Verification items for the finished model (mm, model axes). A direction names the side the tool comes from. Give positions to 0.01 mm unless a question says otherwise; leave off trailing zeros. Order: outer loops, then holes, each group sorted by start corner. A loop starts at its lowest first (then second) coordinate and runs counter-clockwise, first axis right, second up.
from build123d import *

# Parameters (mm, degrees)
SKETCH1_W                      = 60
SKETCH1_H                      = 322.5
BASE_FLANGE1_DEPTH             = 3
EDGE_FLANGE1_STRIP_W           = 14
EDGE_FLANGE1_STRIP_H           = 3
EDGE_FLANGE1_STRIP_CUT_DEPTH   = 322.5
EDGE_FLANGE1_DEPTH             = 322.5
EDGE_FLANGE2_STRIP_W           = 14
EDGE_FLANGE2_STRIP_H           = 3
EDGE_FLANGE2_STRIP_CUT_DEPTH   = 56
EDGE_FLANGE2_STRIP_2_W         = 14
EDGE_FLANGE2_STRIP_2_H         = 3
EDGE_FLANGE2_STRIP_CUT_2_DEPTH = 56
EDGE_FLANGE2_STRIP_3_W         = 14
EDGE_FLANGE2_STRIP_3_H         = 3
EDGE_FLANGE2_STRIP_CUT_3_DEPTH = 56
EDGE_FLANGE2_STRIP_4_W         = 14
EDGE_FLANGE2_STRIP_4_H         = 3
EDGE_FLANGE2_STRIP_CUT_4_DEPTH = 56
EDGE_FLANGE2_DEPTH             = 56
EDGE_FLANGE2_BEND_DEPTH        = 56
EDGE_FLANGE2_BEND_2_DEPTH      = 56
EDGE_FLANGE2_BEND_3_DEPTH      = 56
SKETCH18_R                     = 4.6
EXTRUDE1_DEPTH                 = 335.806287277
SKETCH19_R                     = 4.6
EXTRUDE2_DEPTH                 = 3
SKETCH20_R                     = 4.6
EXTRUDE3_DEPTH                 = 3


# Sheet-metal steps are written as plain solids
with BuildPart() as part:
    # Sketch1 → Base-Flange1 (new body)
    with BuildSketch(Plane(origin=(0, 0, 0), x_dir=(1, 0, 0), z_dir=(0, 1, 0))):
        Rectangle(SKETCH1_W, SKETCH1_H)
    extrude(amount=BASE_FLANGE1_DEPTH)

    # Edge-Flange1 strip (across the edge) → Edge-Flange1 strip cut (cut)
    with BuildSketch(Plane(origin=(-30, 3, -161.25), x_dir=(1, 0, 0), z_dir=(0, 0, 1))):
        with Locations((-3, -1.5)):
            Rectangle(EDGE_FLANGE1_STRIP_W, EDGE_FLANGE1_STRIP_H)
    extrude(amount=EDGE_FLANGE1_STRIP_CUT_DEPTH, mode=Mode.SUBTRACT)

    # Edge-Flange1 section (across the edge) → Edge-Flange1 (add)
    with BuildSketch(Plane(origin=(-30, 3, -161.25), x_dir=(1, 0, 0), z_dir=(0, 0, 1))):
        with BuildLine():
            Line((0, 1), (0, 57))
            Line((0, 57), (3, 57))
            Line((3, 57), (3, 1))
            ThreePointArc((3, 1), (3.292893219, 0.292893219), (4, 0))
            Line((4, 0), (4, -3))
            ThreePointArc((4, -3), (1.171572875, -1.828427125), (0, 1))
        make_face()
    extrude(amount=EDGE_FLANGE1_DEPTH)

    # Edge-Flange2 strip (across the edge) → Edge-Flange2 strip cut (cut)
    with BuildSketch(Plane(origin=(-30, 4, 161.25), x_dir=(0, 0, -1), z_dir=(0, 1, 0))):
        with Locations((-3, -1.5)):
            Rectangle(EDGE_FLANGE2_STRIP_W, EDGE_FLANGE2_STRIP_H)
    extrude(amount=EDGE_FLANGE2_STRIP_CUT_DEPTH, mode=Mode.SUBTRACT)

    # Edge-Flange2 strip 2 (across the edge) → Edge-Flange2 strip cut 2 (cut)
    with BuildSketch(Plane(origin=(30, 0, 161.25), x_dir=(0, 0, -1), z_dir=(-1, 0, 0))):
        with Locations((-3, -1.5)):
            Rectangle(EDGE_FLANGE2_STRIP_2_W, EDGE_FLANGE2_STRIP_2_H)
    extrude(amount=EDGE_FLANGE2_STRIP_CUT_2_DEPTH, mode=Mode.SUBTRACT)

    # Edge-Flange2 strip 3 (across the edge) → Edge-Flange2 strip cut 3 (cut)
    with BuildSketch(Plane(origin=(-30, 60, -161.25), x_dir=(0, 0, 1), z_dir=(0, -1, 0))):
        with Locations((-3, -1.5)):
            Rectangle(EDGE_FLANGE2_STRIP_3_W, EDGE_FLANGE2_STRIP_3_H)
    extrude(amount=EDGE_FLANGE2_STRIP_CUT_3_DEPTH, mode=Mode.SUBTRACT)

    # Edge-Flange2 strip 4 (across the edge) → Edge-Flange2 strip cut 4 (cut)
    with BuildSketch(Plane(origin=(-26, 0, -161.25), x_dir=(0, 0, 1), z_dir=(1, 0, 0))):
        with Locations((-3, -1.5)):
            Rectangle(EDGE_FLANGE2_STRIP_4_W, EDGE_FLANGE2_STRIP_4_H)
    extrude(amount=EDGE_FLANGE2_STRIP_CUT_4_DEPTH, mode=Mode.SUBTRACT)

    # Edge-Flange2 section (across the edge) → Edge-Flange2 (add)
    with BuildSketch(Plane(origin=(-30, 4, 161.25), x_dir=(0, 0, -1), z_dir=(0, 1, 0))):
        with BuildLine():
            Line((0, 1), (0, 37))
            Line((0, 37), (3, 37))
            Line((3, 37), (3, 1))
            ThreePointArc((3, 1), (3.292893219, 0.292893219), (4, 0))
            Line((4, 0), (4, -3))
            ThreePointArc((4, -3), (1.171572875, -1.828427125), (0, 1))
        make_face()
    extrude(amount=EDGE_FLANGE2_DEPTH)

    # Edge-Flange2 section 2 (across the edge) → Edge-Flange2 bend (add)
    with BuildSketch(Plane(origin=(30, 0, 161.25), x_dir=(0, 0, -1), z_dir=(-1, 0, 0))):
        with BuildLine():
            Line((0, 1), (0, 37))
            Line((0, 37), (3, 37))
            Line((3, 37), (3, 1))
            ThreePointArc((3, 1), (3.292893219, 0.292893219), (4, 0))
            Line((4, 0), (4, -3))
            ThreePointArc((4, -3), (1.171572875, -1.828427125), (0, 1))
        make_face()
    extrude(amount=EDGE_FLANGE2_BEND_DEPTH)

    # Edge-Flange2 section 3 (across the edge) → Edge-Flange2 bend 2 (add)
    with BuildSketch(Plane(origin=(-30, 60, -161.25), x_dir=(0, 0, 1), z_dir=(0, -1, 0))):
        with BuildLine():
            Line((0, 1), (0, 37))
            Line((0, 37), (3, 37))
            Line((3, 37), (3, 1))
            ThreePointArc((3, 1), (3.292893219, 0.292893219), (4, 0))
            Line((4, 0), (4, -3))
            ThreePointArc((4, -3), (1.171572875, -1.828427125), (0, 1))
        make_face()
    extrude(amount=EDGE_FLANGE2_BEND_2_DEPTH)

    # Edge-Flange2 section 4 (across the edge) → Edge-Flange2 bend 3 (add)
    with BuildSketch(Plane(origin=(-26, 0, -161.25), x_dir=(0, 0, 1), z_dir=(1, 0, 0))):
        with BuildLine():
            Line((0, 1), (0, 37))
            Line((0, 37), (3, 37))
            Line((3, 37), (3, 1))
            ThreePointArc((3, 1), (3.292893219, 0.292893219), (4, 0))
            Line((4, 0), (4, -3))
            ThreePointArc((4, -3), (1.171572875, -1.828427125), (0, 1))
        make_face()
    extrude(amount=EDGE_FLANGE2_BEND_3_DEPTH)

    # Sketch18 → Extrude1 (cut, through all)
    with BuildSketch(Plane.XY.offset(161.25)):
        with Locations((-47, 47.5)):
            Circle(SKETCH18_R)
        with Locations((-47, 17.5)):
            Circle(SKETCH18_R)
        with Locations((-12.5, -17)):
            Circle(SKETCH18_R)
        with Locations((17.5, -17)):
            Circle(SKETCH18_R)
    extrude(amount=-EXTRUDE1_DEPTH, mode=Mode.SUBTRACT)

    # Sketch19 → Extrude2 (cut)
    with BuildSketch(Plane(origin=(-27, 0, 0), x_dir=(0, 0, -1), z_dir=(1, 0, 0))):
        with Locations(Location((-111.25, 35, 0), (0, 0, 90))):
            Circle(SKETCH19_R)
        with Locations(Location((81.25, 35, 0), (0, 0, 90))):
            Circle(SKETCH19_R)
    extrude(amount=-EXTRUDE2_DEPTH, mode=Mode.SUBTRACT)

    # Sketch20 → Extrude3 (cut)
    with BuildSketch(Plane(origin=(0, 3, 0), x_dir=(1, 0, 0), z_dir=(0, 1, 0))):
        with Locations(Location((5, 81.25, 0), (0, 0, 270))):
            Circle(SKETCH20_R)
        with Locations(Location((5, -111.25, 0), (0, 0, 270))):
            Circle(SKETCH20_R)
    extrude(amount=-EXTRUDE3_DEPTH, mode=Mode.SUBTRACT)


solid = part.part
(1) Section check C-C, the plane x = 17.5. Enter the section's corners in (y, z), then the cut area to 3 significant figures.
Solved:
outline: (-37, -161.25) - (-21.6, -161.25) - (-21.6, -158.25) - (-37, -158.25) - close; (-37, 158.25) - (-21.6, 158.25) - (-21.6, 161.25) - (-37, 161.25) - close; (-12.4, -161.25) - (-1, -161.25) arc R4 ccw to (3, -157.25) - (3, 157.25) arc R4 ccw to (-1, 161.25) - (-12.4, 161.25) - (-12.4, 158.25) - (-1, 158.25) arc R1 cw to (0, 157.25) - (0, -157.25) arc R1 cw to (-1, -158.25) - (-12.4, -158.25) - close
area: 1,130 mm2
(2) Section check A-A, the plane y = 35. Enter the section's corners in (x, z).
Solved:
outline: (-67, -161.25) - (-31, -161.25) arc R4 ccw to (-27, -157.25) - (-27, -85.85) - (-30, -85.85) - (-30, -157.25) arc R1 cw to (-31, -158.25) - (-67, -158.25) - close; (-67, 158.25) - (-31, 158.25) arc R1 cw to (-30, 157.25) - (-30, 115.85) - (-27, 115.85) - (-27, 157.25) arc R4 ccw to (-31, 161.25) - (-67, 161.25) - close; (-30, -76.65) - (-27, -76.65) - (-27, 106.65) - (-30, 106.65) - close
(3) Go/stop test with flat-tipped pins: pin 1 (1 mm diameter, centred on y = 8.5, z = 63.5, fed in from -X); pin 2 (3 mm diameter, centred on x = -53, y = 1.5, fed in from +Z); pin 3 (1.5 mm diameter, centred on x = 13, z = 58, fed in from +Y); pin 4 (1.2 mm diameter, centred on y = -19, z = -159.5, fed in from -X). Record where each tip stops, or that it passes through.
Solved:
pin 1: stops at x = -30
pin 2: passes through
pin 3: stops at y = 3
pin 4: stops at x = -26
(4) Section check B-B, the plane z = 111.25. Enter the section's corners in (x, y), then the cut area to 3 significant figures.
Solved:
outline: (-30, 4) arc R4 ccw to (-26, 0) - (0.4, 0) - (0.4, 3) - (-26, 3) arc R1 cw to (-27, 4) - (-27, 30.4) - (-30, 30.4) - close; (-30, 39.6) - (-27, 39.6) - (-27, 60) - (-30, 60) - close; (9.6, 0) - (30, 0) - (30, 3) - (9.6, 3) - close
area: 293 mm2
(5) Set-up check for faces 1 (the flat face through (2, -19, -158.25)), 2 (the flat face through (-49, 32, 158.25)), 3 (the cylindrical face through (-13.1, -12.44, -159.73)): record each of +Z, -Z, +X, -X, +Y, -Y from which the full face is reachable in a straight line by a thin tool's end or side.
Solved:
face 1: +X, -X, -Y
face 2: -X, +Y, -Y
face 3: +Z, -Z
(6) Release check for a two-part mould opening along Y. For faces 4 (the flat face through (2, 3, -2)), 5 (the cylindrical face through (-28.479, 37.123, 107.169)), 6 (the flat face through (-27, 32, -2)) record: pulls with the +Y half, pulls with the -Y half, needs draft (parallel to the pull), parting line crosses it, or undercut.
Solved:
face 4: pulls with the +Y half
face 5: undercut
face 6: needs draft
(7) Section check D-D, the plane y = -17. Enter the section's corners in (x, z), then the cut area to 3 significant figures.
Solved:
outline: (-26, -161.25) - (-17.1, -161.25) - (-17.1, -158.25) - (-26, -158.25) - close; (-26, 158.25) - (-17.1, 158.25) - (-17.1, 161.25) - (-26, 161.25) - close; (-7.9, -161.25) - (12.9, -161.25) - (12.9, -158.25) - (-7.9, -158.25) - close; (-7.9, 158.25) - (12.9, 158.25) - (12.9, 161.25) - (-7.9, 161.25) - close; (22.1, -161.25) - (30, -161.25) - (30, -158.25) - (22.1, -158.25) - close; (22.1, 158.25) - (30, 158.25) - (30, 161.25) - (22.1, 161.25) - close
area: 226 mm2
(8) Scan lines: line 1 (Z direction, x = -36, y = 46.5); line 2 (X direction, y = 8, z = 148); line 3 (Y direction, x = 25.5, z = 100). Record each from-to range of solid material in increasing order.
Solved:
line 1: z = -161.25 to -158.25, 158.25 to 161.25
line 2: x = -30 to -27
line 3: y = 0 to 3
